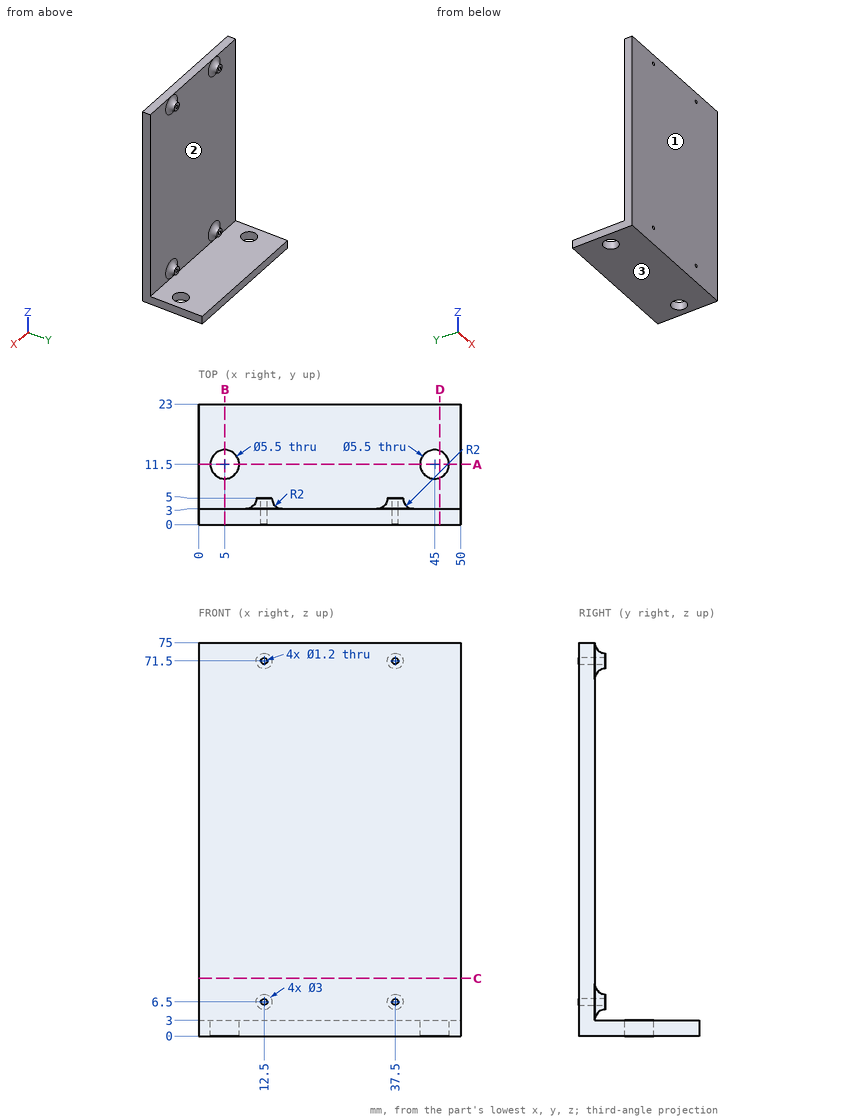
The drawing under review shows one solid part. Ordinate dimensions are in mm from its lowest x, y, z. Coordinates: 2 decimals unless noted, no trailing zeros. Order: outer loops, then holes, each group sorted by start corner. A loop starts at its lowest first (then second) coordinate and runs counter-clockwise, first axis right, second up. Notation, with made-up numbers: (60.5, 29.5) -> (74.5, 29.5) arc R20 cw to (74.5, 46.5) -> close; hole circle Ø9 at (81.5, 15.5). An arc over 180 degrees is marked (long way). Return JSON: item names as keys, results as strings.
1. We need section C-C on z = 11. Write out the cut boundary in (x, y).
Answer block:
{"outline": "(0, 0) -> (50, 0) -> (50, 3) -> (0, 3) -> close"}
2. The part is to be moulded in two halves that separate along Z. For the marked faces 1, 2 and 3, say which applies: +Z half, -Z half, draft (parallel to the pull), parting line (faces both ways), or undercut.
Answer block:
{"face 1": "draft", "face 2": "undercut", "face 3": "-Z half"}
3. For pin 1 Ø1 at (x, z) = (37.5, 6.5) entering from +Y; pin 2 Ø3.5 at (x, z) = (13, 6.5) entering from +Y; pin 3 Ø7 at (x, y) = (5, 11.5) entering from +Z; pin 4 Ø6 at (x, z) = (27.5, 15.5) entering from +Y, all flat-tipped, find the tip position at first contact; note any pin that passes through.
Answer block:
{"pin 1": "through", "pin 2": "y = 5", "pin 3": "z = 3", "pin 4": "y = 3"}
4. We need section D-D on x = 46. Write out the cut boundary in (y, z).
Answer block:
{"outline": "(0, 0) -> (8.94, 0) -> (8.94, 3) -> (3, 3) -> (3, 75) -> (0, 75) -> close; (14.06, 0) -> (23, 0) -> (23, 3) -> (14.06, 3) -> close"}
5. We need section B-B on x = 5. Write out the cut boundary in (y, z).
Answer block:
{"outline": "(0, 0) -> (8.75, 0) -> (8.75, 3) -> (3, 3) -> (3, 75) -> (0, 75) -> close; (14.25, 0) -> (23, 0) -> (23, 3) -> (14.25, 3) -> close"}
6. We need section A-A on y = 11.5. Write out the cut boundary in (x, z), and give its area (3 significant figures).
Answer block:
{"outline": "(0, 0) -> (2.25, 0) -> (2.25, 3) -> (0, 3) -> close; (7.75, 0) -> (42.25, 0) -> (42.25, 3) -> (7.75, 3) -> close; (47.75, 0) -> (50, 0) -> (50, 3) -> (47.75, 3) -> close", "area": "117 mm²"}
7. For line 1 (X direction, y = 2, z = 71.5); line 2 (Z direction, x = 37.5, y = 2.35); line 3 (Y direction, x = 22, z = 8), list the stretches that pass through material, from the lowest coordinate up. Write a range as from..to.
Answer block:
{"line 1": "0..11.9, 13.1..36.9, 38.1..50", "line 2": "0..5.9, 7.1..70.9, 72.1..75", "line 3": "0..3"}
